Job drawing, mm, ordinate dimensions from the low corner. One solid piece. Coordinates: 2 decimals unless noted, no trailing zeros. Loops run counter-clockwise (first coordinate to the right, second up) from the corner with the lowest first, then second, coordinate; pieces in that order, holes last. Notation, with made-up numbers: (26, 65) -> (76, 65) arc R11 ccw to (76, 74) -> close; hole circle Ø4 at (55.5, 65). An arc over 180 degrees is marked (long way). Answer as CSV lines item,"result". Start each with the question number.
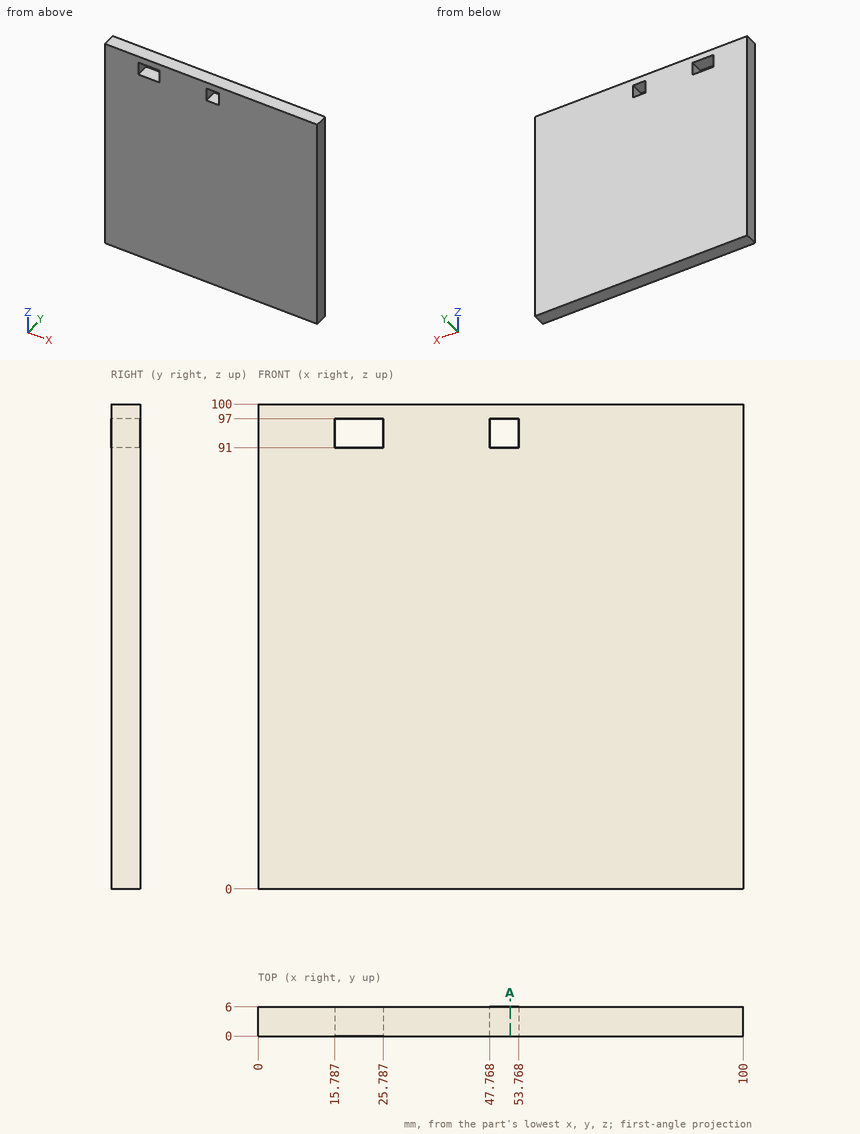
Q1. Pin check, flat tip, straight feed: pin 1 Ø3 at (x, y) = (49.5, 2.5) entering from -Z. Stop position of the tip, or through.
Q2. Saw through at A-A (x = 52). List the corners of the cut face in (y, z), and give its area (3 significant figures).
Q3. Probe probe 1 along X at (y, z) = (2.8, 95); probe 2 along Z at (x, y) = (16, 4.25). List the from-to ranges inside material, lowest first. Write a range as from..to.
Ans:
1,pin 1,"stops at z = 0"
2,outline,"(0, 0) -> (6, 0) -> (6, 91) -> (0, 91) -> close; (0, 97) -> (6, 97) -> (6, 100) -> (0, 100) -> close"
2,area,"564 mm²"
3,probe 1,"x = 0..15.79, 25.79..47.77, 53.77..100"
3,probe 2,"z = 0..91, 97..100"
